Source: CAD feature listing. Evaluate the final solid. Frame: model axes, mm. A direction names the side the tool comes from. Round coordinates to 2 decimals unless told otherwise and drop trailing zeros. Order: outer loops, then holes, each group sorted by start corner. A loop starts at its lowest first (then second) coordinate and runs counter-clockwise, first axis right, second up. Notation, with made-up numbers: (37.5, -9.75) - (47.5, -9.75) arc R10 ccw to (47.5, 0.25) - close; hole circle Ø3 at (64.5, 74). An arc over 180 degrees is marked (long way). Put each result on its own line as item: value. Start each with the question number.
1) Line query: probe 1 along Y at (x, z) = (126.9, 0); probe 2 along X at (y, z) = (22, 11); probe 3 along X at (y, z) = (-18, -15). Output: solid intervals per line, ascending. Write a range as [from, to].
2) Section C-C on x = 16. Output: boundary loops of the cut face in (y, z).
3) Mould query, pull axis Z, two halves, no side actions, for faces 1 (the face through (45.1, -19.6, 4.3)), 2 (the face through (17.78, 22, 0)), 3 (the face through (113.538, 0, 19)). Classes: +Z half, -Z half, draft (parallel to the pull), parting line (faces both ways), or undercut.
4) Section A-A on y = 21.5. Output: boundary loops of the cut face in (x, z), then the cut area to 3 significant figures.
5) Section D-D on y = -17.5. Output: boundary loops of the cut face in (x, z).
6) Contact query for flat-ended pins moving along their axis: P1, Ø5.5, axis at x = 13, y = 15, coming from the -Z side; P2, Ø3, axis at x = 124, z = -15.5, coming from the +Y side; P3, Ø14.5, axis at y = 2.5, z = -6, coming from the +X side. Output: stop coordinate, or through.
7) Access query for faces 4 (the face through (145.796, -8, 0)), 5 (the face through (108.6, -24.77, 5.5)), 6 (the face through (91.44, 8, -19)), 7 (the face through (9, 26.162, 0)), 8 (the face through (9, 13, -20.066)). Directions: +Z, -Z, +X, -X, +Y, -Y. A direction counts if a zero-diameter tool reaches every point of the face in a straight line with its end or side. Return the directions, or none.
8) Section B-B on z = 0. Output: boundary loops of the cut face in (x, y), then the cut area to 3 significant figures.
```python
from build123d import *

# Parameters (mm, degrees)
SKETCH1_R           = 20.066
BOSS_EXTRUDE1_DEPTH = 91.44
BOSS_EXTRUDE2_DEPTH = 17.78
SKETCH3_R           = 25.3746
BOSS_EXTRUDE3_DEPTH = 34.798
SKETCH5_R           = 14.2748
SKETCH5_R_2         = 4.7625
BOSS_EXTRUDE5_DEPTH = 1.524
SKETCH6_R           = 3.175
BOSS_EXTRUDE6_DEPTH = 19.558
SKETCH7_R           = 2.3876
CUT_EXTRUDE1_DEPTH  = 12.7


with BuildPart() as part:
    # Sketch1 → Boss-Extrude1 (new body)
    with BuildSketch(Plane(origin=(0, 0, 0), x_dir=(0, 0, -1), z_dir=(1, 0, 0))):
        Circle(SKETCH1_R)
    extrude(amount=BOSS_EXTRUDE1_DEPTH)

    # Sketch2 → Boss-Extrude2 (add)
    with BuildSketch(Plane.ZY):
        with BuildLine():
            Line((-20.066, 26.162), (20.066, 26.162))
            Line((20.066, 26.162), (20.066, 0))
            ThreePointArc((20.066, 0), (0, -20.066), (-20.066, 0))
            Line((-20.066, 0), (-20.066, 26.162))
        make_face()
    extrude(amount=-BOSS_EXTRUDE2_DEPTH)

    # Sketch3 → Boss-Extrude3 (add)
    with BuildSketch(Plane(origin=(91.44, 0, 0), x_dir=(0, 0, -1), z_dir=(1, 0, 0))):
        Circle(SKETCH3_R)
    extrude(amount=BOSS_EXTRUDE3_DEPTH)

    # Sketch5 → Boss-Extrude5 (add)
    with BuildSketch(Plane(origin=(126.238, 0, 0), x_dir=(0, 0, -1), z_dir=(1, 0, 0))):
        with Locations(Location((0, 0, 0), (0, 0, 180))):
            Circle(SKETCH5_R)
        with Locations(Location((0, -8.2296, 0), (0, 0, 180))):
            Circle(SKETCH5_R_2, mode=Mode.SUBTRACT)
    extrude(amount=BOSS_EXTRUDE5_DEPTH)

    # Sketch6 → Boss-Extrude6 (add)
    with BuildSketch(Plane(origin=(126.238, 0, 0), x_dir=(0, 0, -1), z_dir=(1, 0, 0))):
        with Locations((0, -8.2296)):
            Circle(SKETCH6_R)
    extrude(amount=BOSS_EXTRUDE6_DEPTH)

    # Sketch7 → Cut-Extrude1 (cut)
    with BuildSketch(Plane(origin=(126.238, 0, 0), x_dir=(0, 0, -1), z_dir=(1, 0, 0))):
        with Locations((18.7833, 0)):
            Circle(SKETCH7_R)
        with Locations(Location((-18.7833, 0, 0), (0, 0, 180))):
            Circle(SKETCH7_R)
    extrude(amount=-CUT_EXTRUDE1_DEPTH, mode=Mode.SUBTRACT)


solid = part.part
```
Answer sheet:
1. probe 1: [-14.27, -12.99], [-11.4, -5.05], [-3.47, 14.27]
1. probe 2: [0, 17.78], [91.44, 126.24]
1. probe 3: [91.44, 126.24]
2. outline: (0, -20.07) - (26.16, -20.07) - (26.16, 20.07) - (0, 20.07) arc R20.07 ccw to start
3. face 1: parting line
3. face 2: draft
3. face 3: undercut
4. outline: (0, -20.07) - (17.78, -20.07) - (17.78, 20.07) - (0, 20.07) - close; (91.44, -13.48) - (126.24, -13.48) - (126.24, 13.48) - (91.44, 13.48) - close
4. area: 1,650 mm^2
5. outline: (0, -9.82) - (91.44, -9.82) - (91.44, -18.37) - (126.24, -18.37) - (126.24, 18.37) - (91.44, 18.37) - (91.44, 9.82) - (0, 9.82) - close
6. P1: z = -20.07
6. P2: y = 21.16
6. P3: x = 127.76
7. face 4: +Z, -Z, +X, +Y, -Y
7. face 5: +X
7. face 6: none
7. face 7: +Z, -Z, +X, -X, +Y
7. face 8: -Z, -X, +Y, -Y
8. outline: (0, -20.07) - (91.44, -20.07) - (91.44, -25.37) - (126.24, -25.37) - (126.24, -14.27) - (127.76, -14.27) - (127.76, -12.99) - (126.24, -12.99) - (126.24, -11.4) - (145.8, -11.4) - (145.8, -5.05) - (126.24, -5.05) - (126.24, -3.47) - (127.76, -3.47) - (127.76, 14.27) - (126.24, 14.27) - (126.24, 25.37) - (91.44, 25.37) - (91.44, 20.07) - (17.78, 20.07) - (17.78, 26.16) - (0, 26.16) - close
8. area: 5,700 mm^2
